Can you work these out from the model? Positions are in its coordinate system, mm. Face numbers are marked on the shaded views. A direction names the side the tool comes from. Give positions to 0.01 mm unless a question says otherwise; leave off trailing zeros. Write each loop counter-clockwise with the first axis right and the second up, starting at its lowest first coordinate (ties: lowest second). Pieces come first, ordered by that corner, then holes.
1. Suppose I cut it at A-A (z = -9.5). Please give me the cut outline in (x, y), and give its area (3 significant figures).
2. On a 3-axis mill with a long thin cutter (end or side, diameter ignored), from which of +Z, -Z, +X, -X, +Y, -Y can I reach the whole of each face in a straight line? I mean the marked faces 1, 2 and 3. Say none if no direction works.
3. If I drill on probe 1 along Y at (x, z) = (0, 26); probe 2 along X at (y, z) = (-18, 11.5); probe 3 along Y at (x, z) = (13.5, 14.5), over which ranges is the centre line in solid material (lowest first)?
4. Suppose I cut it at B-B (z = 5). Please give me the cut outline in (x, y).
5. I'm going to push flat-ended pins straight in: pin 1 (12 mm diameter, centred on x = -0.5, y = -3, fed in from -Z); pin 2 (1.5 mm diameter, centred on x = -10, y = -17, fed in from +Z); pin 3 (4.5 mm diameter, centred on x = 1.5, y = -27, fed in from +Z). Where does each tip first touch, or does it pass through?
6. Suppose I cut it at C-C (y = 0). Please give me the cut outline in (x, z), and give its area (3 significant figures).
7. Suppose I cut it at D-D (y = 16.5). Please give me the cut outline in (x, z), and give its area (3 significant figures).
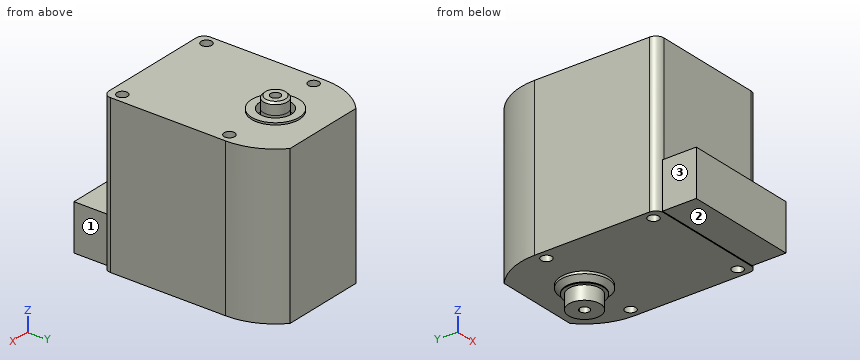
Autodesk Inventor part; units mm, degrees
ref_plane "YZ Plane" through (0, 0, 0) normal (1, 0, 0) x (0, 1, 0)
ref_plane "XZ Plane" through (0, 0, 0) normal (0, 1, 0) x (-1, 0, 0)
ref_plane "XY Plane" through (0, 0, 0) normal (0, 0, 1) x (1, 0, 0)
sketch "スケッチ1" plane through (0, 0, 0) normal (0, 0, 1) x (1, 0, 0)
  line L0 (-16, 21.5) -> (-10.583, 21.5) construction
  line L1 (16, 21.5) -> (16, 9.5) construction
  line L2 (16, -21.5) -> (-16, -21.5)
  line L3 (-16, -21.5) -> (-16, 9.5)
  line L4 (-16, 21.5) -> (16, -21.5) construction
  line L5 (16, 21.5) -> (-16, -21.5) construction
  line L6 (-14.4, -21.5) -> (-14.4, -30)
  line L7 (-14.4, -30) -> (14.4, -30)
  line L8 (0, 21.5) -> (0, -21.5) construction
  line L9 (14.4, -21.5) -> (14.4, -30)
  line L10 (-13.5, 21.5) -> (-13.5, -21.5) construction
  circle A0 centre (0, 9.5) radius 6
  circle A1 centre (0, 9.5) radius 4
  arc A2 (-10.583, 21.5) -> (-16, 9.5) centre (0, 9.5) ccw
  arc A3 (16, 9.5) -> (10.583, 21.5) centre (0, 9.5) ccw
  line L11 (-10.583, 21.5) -> (10.583, 21.5)
  line L12 (-16, 9.5) -> (-16, 21.5) construction
  line L13 (10.583, 21.5) -> (16, 21.5) construction
  line L14 (16, 9.5) -> (16, -21.5)
  circle A4 centre (0, 9.5) radius 3
  circle A5 centre (0, 9.5) radius 4.8
  point P0 (0, 0)
  point P1 (-13.5, 8.5)
  point P2 (-13.5, -18.5)
  point P3 (13.5, 8.5)
  point P4 (13.5, -18.5)
  dimension "d0" = 32
  dimension "d1" = 43
  dimension "d4" = 28.8
  dimension "d5" = 8.5
  dimension "d8" = 27
  dimension "d9" = 8.5
  dimension "d12" = 18.5
  dimension "d13" = 12
  dimension "d14" = 8
  dimension "d15" = 9.5
  dimension "d17" = 16
  dimension "d32" = 13.5
  dimension "d47" = 6
  dimension "d67" = 9.6
extrude "押し出し1" add sketch "スケッチ1" against normal blind 12.2 contours L2 L3 A2 L11 A3 L14 | A0 | A1 | A4 | A5
extrude "押し出し2" add sketch "スケッチ1" against normal blind 12 contours L9 L7 L6 L2
extrude "押し出し3" add sketch "スケッチ1" against normal blind 14 contours A0 | A1 | A4 | A5
extrude "押し出し4" add sketch "スケッチ1" against normal blind 17.7 contours A1 | A4
chamfer "面取り1" distance 1.2 angle 45 1 edges at (-6, 9.5, -14)
sketch "スケッチ2" plane through (0, 9.5, -17.7) normal (0, 0, -1) x (-1, 0, 0)
  circle A0 centre (0, 0) radius 4
  point P0 (0, -9.5)
hole "穴1" at (0, 9.5, -17.7) direction (0, 0, 1) diameter 2.459 depth 6
extrude "押し出し5" add sketch "スケッチ1" along normal blind 27.3 contours L2 L3 A2 L11 A3 L14 | A0 | A1 | A4 | A5
hole "穴2" at (-13.5, 8.5, 0) at (-13.5, -18.5, 0) at (13.5, 8.5, 0) at (13.5, -18.5, 0) direction (0, 0, 1) diameter 2.7 end through all both
extrude "押し出し6" cut sketch "スケッチ1" against normal blind 0.4 contours L9 L7 L6 L2
fillet "フィレット1" radius 2 2 edges at (16, -21.5, 7.55) (-16, -21.5, 7.55)
extrude "押し出し7" add sketch "スケッチ1" along normal blind 27.8 contours A0 | A1 | A4 | A5
extrude "押し出し8" add sketch "スケッチ1" along normal blind 30.75 contours A4
sketch "スケッチ3" plane through (0, 9.5, 30.75) normal (0, 0, 1) x (1, 0, 0)
  circle A0 centre (0, 0) radius 1.2295
  point P0 (0, -9.5)
hole "穴3" at (0, 9.5, 30.75) direction (0, 0, -1) diameter 2.459 end through all
sketch "スケッチ4" plane through (0, 9.5, 27.8) normal (0, 0, 1) x (1, 0, 0)
  circle A0 centre (0, 0) radius 4
  circle A1 centre (0, 0) radius 3
  point P0 (0, -9.5)
extrude "押し出し9" cut sketch "スケッチ4" against normal blind 2.3
chamfer "面取り2" distance 0.5 angle 45 1 edges at (-3, 9.5, 30.75)
extrude "押し出し10" add sketch "スケッチ1" against normal blind 14.2 contours A5
properties part number "B3M11xx"
Checks:
1. outline: (-16, -19.5) arc R2 ccw to (-14.4, -21.46) - (-14.4, -30) - (14.4, -30) - (14.4, -21.46) arc R2 ccw to (16, -19.5) - (16, 9.5) arc R16 ccw to (10.58, 21.5) - (-10.58, 21.5) arc R16 ccw to (-16, 9.5) - close; hole circle Ø2.7 at (-13.5, -18.5); hole circle Ø2.7 at (-13.5, 8.5); hole circle Ø2.46 at (0, 9.5); hole circle Ø2.7 at (13.5, -18.5); hole circle Ø2.7 at (13.5, 8.5)
1. area: 1,550 mm2
2. face 1: +Z, -Z, +X, -Y
2. face 2: -Z, +X, -X, -Y
2. face 3: +Z, -Z, -X, -Y
3. probe 1: y = -21.5 to 5.5, 6.5 to 8.27, 10.73 to 12.5, 13.5 to 21.5
3. probe 2: x = -16 to -14.75, -12.25 to 12.25, 14.75 to 16
3. probe 3: y = -21.5 to -19.85, -17.15 to 7.15, 9.85 to 18.09
4. outline: (-16, -19.5) arc R2 ccw to (-14, -21.5) - (14, -21.5) arc R2 ccw to (16, -19.5) - (16, 9.5) arc R16 ccw to (10.58, 21.5) - (-10.58, 21.5) arc R16 ccw to (-16, 9.5) - close; hole circle Ø2.7 at (-13.5, -18.5); hole circle Ø2.7 at (-13.5, 8.5); hole circle Ø2.46 at (0, 9.5); hole circle Ø2.7 at (13.5, -18.5); hole circle Ø2.7 at (13.5, 8.5)
5. pin 1: stops at z = -12.2
5. pin 2: stops at z = 27.3
5. pin 3: stops at z = -0.4
6. outline: (-16, -12.2) - (16, -12.2) - (16, 27.3) - (-16, 27.3) - close
6. area: 1,260 mm2
7. outline: (-14.39, -12.2) - (14.39, -12.2) - (14.39, 27.3) - (-14.39, 27.3) - close
7. area: 1,140 mm2
